from build123d import *

# Parameters (mm, degrees)
SKETCH1_W           = 118
SKETCH1_H           = 118
SKETCH1_R           = 4.5
BOSS_EXTRUDE1_DEPTH = 9.85
SKETCH2_R           = 2
CUT_EXTRUDE1_DEPTH  = 5
FILLET1_R           = 21
CHAMFER1_SIZE       = 2
CHAMFER1_SIZE2      = 0.649839392
CHAMFER2_SIZE       = 3
CHAMFER2_SIZE2      = 0.974759089
CHAMFER3_SIZE       = 2


with BuildPart() as part:
    # Sketch1 → Boss-Extrude1 (new body)
    with BuildSketch(Plane(origin=(0, 0, 0), x_dir=(1, 0, 0), z_dir=(0, 1, 0))):
        Rectangle(SKETCH1_W, SKETCH1_H)
        with Locations(Location((0, 0, 0), (0, 0, 270))):
            Circle(SKETCH1_R, mode=Mode.SUBTRACT)
    extrude(amount=BOSS_EXTRUDE1_DEPTH)

    # Sketch2 → Cut-Extrude1 (cut)
    with BuildSketch(Plane(origin=(0, 9.85, 0), x_dir=(1, 0, 0), z_dir=(0, 1, 0))):
        with Locations(Location((0, -48, 0), (0, 0, 270))):
            Circle(SKETCH2_R)
        with Locations(Location((11, -48, 0), (0, 0, 270))):
            Circle(SKETCH2_R)
        with Locations(Location((33, -48, 0), (0, 0, 270))):
            Circle(SKETCH2_R)
        with Locations(Location((-33, -48, 0), (0, 0, 90))):
            Circle(SKETCH2_R)
        with Locations(Location((-11, -48, 0), (0, 0, 90))):
            Circle(SKETCH2_R)
        with Locations(Location((0, -11, 0), (0, 0, 270))):
            Circle(SKETCH2_R)
        with Locations(Location((11, -11, 0), (0, 0, 270))):
            Circle(SKETCH2_R)
        with Locations(Location((-11, -11, 0), (0, 0, 90))):
            Circle(SKETCH2_R)
        with Locations(Location((-11, 0, 0), (0, 0, 270))):
            Circle(SKETCH2_R)
        with Locations(Location((-11, 11, 0), (0, 0, 270))):
            Circle(SKETCH2_R)
        with Locations(Location((11, 11, 0), (0, 0, 90))):
            Circle(SKETCH2_R)
        with Locations(Location((0, 11, 0), (0, 0, 90))):
            Circle(SKETCH2_R)
        with Locations(Location((-11, 48, 0), (0, 0, 270))):
            Circle(SKETCH2_R)
        with Locations(Location((-33, 48, 0), (0, 0, 270))):
            Circle(SKETCH2_R)
        with Locations(Location((33, 48, 0), (0, 0, 90))):
            Circle(SKETCH2_R)
        with Locations(Location((11, 48, 0), (0, 0, 90))):
            Circle(SKETCH2_R)
        with Locations(Location((0, 48, 0), (0, 0, 90))):
            Circle(SKETCH2_R)
        with Locations(Location((11, 0, 0), (0, 0, 90))):
            Circle(SKETCH2_R)
        with Locations(Location((48, 11, 0), (0, 0, 270))):
            Circle(SKETCH2_R)
        with Locations(Location((48, 33, 0), (0, 0, 270))):
            Circle(SKETCH2_R)
        with Locations(Location((48, -33, 0), (0, 0, 90))):
            Circle(SKETCH2_R)
        with Locations(Location((48, -11, 0), (0, 0, 90))):
            Circle(SKETCH2_R)
        with Locations(Location((48, 0, 0), (0, 0, 90))):
            Circle(SKETCH2_R)
        with Locations(Location((-48, 0, 0), (0, 0, 270))):
            Circle(SKETCH2_R)
        with Locations(Location((-48, -11, 0), (0, 0, 270))):
            Circle(SKETCH2_R)
        with Locations(Location((-48, -33, 0), (0, 0, 270))):
            Circle(SKETCH2_R)
        with Locations(Location((-48, 33, 0), (0, 0, 90))):
            Circle(SKETCH2_R)
        with Locations(Location((-48, 11, 0), (0, 0, 90))):
            Circle(SKETCH2_R)
    extrude(amount=-CUT_EXTRUDE1_DEPTH, mode=Mode.SUBTRACT)

    # Fillet1
    fillet1_edges = [part.edges().sort_by_distance(p)[0] for p in [
        (59, 4.925, 59),
        (-59, 4.925, 59),
        (-59, 4.925, -59),
        (59, 4.925, -59),
    ]]
    fillet(fillet1_edges, radius=FILLET1_R)

    # Chamfer1
    chamfer1_edges = [part.edges().sort_by_distance(p)[0] for p in [
        (0, 0, -59),
        (59, 0, 0),
        (0, 0, 59),
        (-59, 0, 0),
        (52.849242405, 0, 52.849242405),
        (-52.849242405, 0, 52.849242405),
        (-52.849242405, 0, -52.849242405),
        (52.849242405, 0, -52.849242405),
    ]]
    chamfer1_side = [part.faces().sort_by_distance(p)[0] for p in [
        (0, 0, 57.331227996),
    ]]
    chamfer(chamfer1_edges, length=CHAMFER1_SIZE, length2=CHAMFER1_SIZE2, reference=chamfer1_side[0])

    # Chamfer2
    chamfer2_edges = [part.edges().sort_by_distance(p)[0] for p in [
        (0, 9.85, -59),
        (59, 9.85, 0),
        (-59, 9.85, 0),
        (0, 9.85, 59),
        (52.849242405, 9.85, 52.849242405),
        (-52.849242405, 9.85, 52.849242405),
        (-52.849242405, 9.85, -52.849242405),
        (52.849242405, 9.85, -52.849242405),
    ]]
    chamfer2_side = [part.faces().sort_by_distance(p)[0] for p in [
        (0, 9.85, 57.331227996),
    ]]
    chamfer(chamfer2_edges, length=CHAMFER2_SIZE, length2=CHAMFER2_SIZE2, reference=chamfer2_side[0])

    # Chamfer3
    chamfer3_edges = [part.edges().sort_by_distance(p)[0] for p in [
        (-50.727922061, 9.85, 50.727922061),
        (0, 9.85, 56),
        (-56, 9.85, 0),
        (50.727922061, 9.85, 50.727922061),
        (-50.727922061, 9.85, -50.727922061),
        (56, 9.85, 0),
        (0, 9.85, -56),
        (50.727922061, 9.85, -50.727922061),
    ]]
    chamfer(chamfer3_edges, length=CHAMFER3_SIZE)


solid = part.part
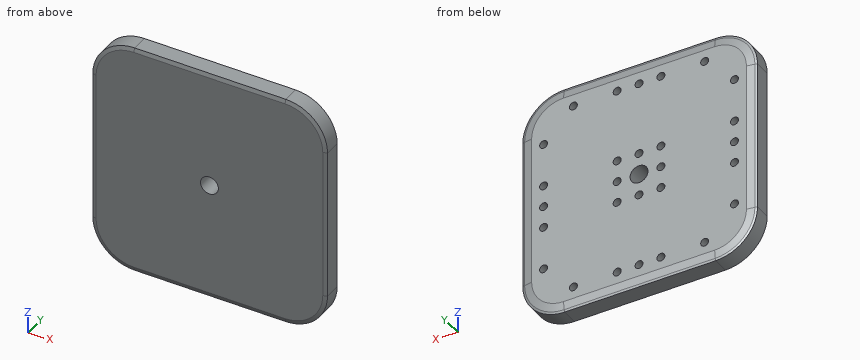
The model under review builds one solid part; all positions refer to its coordinate system, in mm. Round coordinates to 2 decimals unless told otherwise and drop trailing zeros. Loops run counter-clockwise (first coordinate to the right, second up) from the corner with the lowest first, then second, coordinate; pieces in that order, holes last. Notation, with made-up numbers: M -5.75,88 L 6.25,88 A14 ccw 6.25,104 Z; hole C 81.25,37 d8. An arc over 180 degrees is marked long. Answer as a JSON object with one key per item and string values.
Item 1: We need section C-C, the plane y = 2. State the section outline as (x, z) points.
Check sheet entries:
{"outline": "M -59,-38 A21 ccw -38,-59 L 38,-59 A21 ccw 59,-38 L 59,38 A21 ccw 38,59 L -38,59 A21 ccw -59,38 Z; hole C 0,0 d9"}
Item 2: Clearance check with a flat-ended pin moving along its axis: P1, Ø1.2, axis at x = -11, z = 0, coming from the +Y side. State where the tip first meets the part, or that it passes through.
Check sheet entries:
{"P1": "y = 4.85"}
Item 3: For line 1 along X through (y, z) = (7.5, 0); line 2 along X through (y, z) = (8.25, 33); line 3 along X through (y, z) = (5.95, 11), list the stretches that pass through material, from the lowest coordinate up.
Check sheet entries:
{"line 1": "-59 to -50, -46 to -13, -9 to -4.5, 4.5 to 9, 13 to 46, 50 to 59", "line 2": "-59 to -50, -46 to 46, 50 to 59", "line 3": "-59 to -50, -46 to -13, -9 to -2, 2 to 9, 13 to 46, 50 to 59"}
Item 4: We need section A-A, the plane x = -33. State the section outline as (y, z) points, and give its area (3 significant figures).
Check sheet entries:
{"outline": "M 0,-57 L 0.65,-59 L 8.88,-59 L 9.23,-57.9 L 9.85,-54 L 9.85,-50 L 4.85,-50 L 4.85,-46 L 9.85,-46 L 9.85,46 L 4.85,46 L 4.85,50 L 9.85,50 L 9.85,54 L 9.23,57.9 L 8.88,59 L 0.65,59 L 0,57 Z", "area": "1,120 mm2"}
